For this review, take the finished solid that the model builds, in its own axes (mm). A direction names the side the tool comes from. Coordinates: 2 decimals unless noted, no trailing zeros. Order: outer loops, then holes, each group sorted by start corner. A loop starts at its lowest first (then second) coordinate and runs counter-clockwise, first axis right, second up. Notation, with made-up numbers: (81, -19) -> (138, -19) arc R33 cw to (138, 11) -> close; hole circle Ø2 at (65, 42.5). An arc over 180 degrees is marked (long way). Write item = value, one per line. Start each with the question number.
1) Insertion check: pin 1 Ø5 at (x, y) = (-81, 1) entering from -Z; pin 2 Ø3 at (y, z) = (27, 20) entering from +X; pin 3 Ø12.5 at (x, z) = (-18, 10) entering from +Y. Each pin has a flat end and moves straight along its axis. Give the tip position at first contact, or say it passes through.
2) Draft analysis for pull direction Z (two halves, no side actions). For faces 1 (the face through (-153.774, 16.355, 5.948)), 2 (the face through (-106.21, 14.37, 14.76)), 3 (the face through (12.697, -1.252, 12.979)), 4 (the face through (-49, -2.54, 13)), state which applies: +Z half, -Z half, draft (parallel to the pull), parting line (faces both ways), or undercut.
3) Machinability: for faces 5 (the face through (-153.61, 16.35, 21.36)), 6 (the face through (-103.632, 16, 17)), 7 (the face through (-71, -1, 0)), 8 (the face through (-108.712, 15, 10)), 9 (the face through (-156.11, 15.9, 22.45)), which of the approach directions +Z, -Z, +X, -X, +Y, -Y give a long, thin tool a straight path to every point of the face, cutting with its end or side? Answer none if there is none.
4) Consider section A-A on z = 3. Give the boundary of the cut face in (x, y), and give its area (3 significant figures).
5) Consider section C-C on x = -94. Give the boundary of the cut face in (y, z), and give its area (3 significant figures).
6) Wall thickness on probe 1 along Y at (x, z) = (-106.7, 12.7); probe 2 along X at (y, z) = (-1.15, 12.7); probe 3 along Y at (x, z) = (-83, 4.5): over which ranges is each line inside the solid? List them lowest first. Write a range as [from, to].
7) Consider section B-B on x = -131. Give the boundary of the cut face in (y, z), and give its area (3 significant figures).
from build123d import *

# Parameters (mm, degrees)
SKETCH1_R                   = 4.064
BOSS_EXTRUDE1_DEPTH         = 2.54
SKETCH2_W                   = 30.48
SKETCH2_H                   = 32.258
BOSS_EXTRUDE2_DEPTH         = 5.08
SKETCH3_W                   = 41.91
SKETCH3_H                   = 32.258
BOSS_EXTRUDE3_DEPTH         = 2.54
FILLET1_SIZE                = 2.54
CUT_EXTRUDE1_DEPTH          = 158.565599432
SKETCH5_W                   = 17.78
SKETCH5_H                   = 32.258
BOSS_EXTRUDE4_DEPTH         = 2.54
BOSS_EXTRUDE5_DEPTH         = 32.258
SKETCH9_W                   = 18.796
SKETCH9_H                   = 32.258
BOSS_EXTRUDE6_DEPTH         = 2.54
BOSS_EXTRUDE7_DEPTH         = 32.258
FILLET3_SIZE                = 2.54
W_0_22_DIAMETER_HOLE1_D     = 5.588
W_0_22_DIAMETER_HOLE1_DEPTH = 5.08
W_0_22_DIAMETER_HOLE1_TIP   = 1.67880457


with BuildPart() as part:
    # Sketch1 → Boss-Extrude1 (new body)
    with BuildSketch(Plane(origin=(0, 0, 0), x_dir=(1, 0, 0), z_dir=(0, 1, 0))):
        with BuildLine():
            Line((0, 0), (-108.712, 0))
            Line((-108.712, 0), (-108.712, -25.4))
            Line((-108.712, -25.4), (0, -25.4))
            ThreePointArc((0, -25.4), (12.7, -12.7), (0, 0))
        make_face()
        with Locations(Location((0, -12.7, 0), (0, 0, 270))):
            Circle(SKETCH1_R, mode=Mode.SUBTRACT)
    extrude(amount=-BOSS_EXTRUDE1_DEPTH)

    # Sketch2 → Boss-Extrude2 (add)
    with BuildSketch(Plane(origin=(-108.712, 0, 0), x_dir=(0, 0, -1), z_dir=(1, 0, 0))):
        with Locations((-15.24, 16.129)):
            Rectangle(SKETCH2_W, SKETCH2_H)
    extrude(amount=BOSS_EXTRUDE2_DEPTH)

    # Sketch3 → Boss-Extrude3 (add)
    with BuildSketch(Plane.XY.offset(30.48)):
        with Locations((-129.667, 16.129)):
            Rectangle(SKETCH3_W, SKETCH3_H)
    extrude(amount=-BOSS_EXTRUDE3_DEPTH)

    # Fillet1
    # a fillet whose section is not a circle: 2.54 mm, written as the material it adds along each edge
    with BuildSketch(Plane(origin=(-108.712, 0, 27.94), x_dir=(0, 0, -1), z_dir=(0, 1, 0))) as fillet1_piece_1:
        with BuildLine():
            Bezier((FILLET1_SIZE, 0), (0, 0), (0, FILLET1_SIZE), weights=[1, 1, 1])
            Line((0, FILLET1_SIZE), (0, 0))
            Line((0, 0), (FILLET1_SIZE, 0))
        make_face()
    extrude(amount=32.258)
    # a fillet whose section is not a circle: 2.54 mm, written as the material it takes off along each edge
    with BuildSketch(Plane(origin=(-103.632, -6.35, 30.48), x_dir=(0, 0, -1), z_dir=(0, 1, 0))) as fillet1_2_piece_1:
        with BuildLine():
            Bezier((FILLET1_SIZE, 0), (0, 0), (0, FILLET1_SIZE), weights=[1, 1, 1])
            Line((0, FILLET1_SIZE), (0, 0))
            Line((0, 0), (FILLET1_SIZE, 0))
        make_face()
    extrude(amount=44.958, mode=Mode.SUBTRACT)

    # Sketch4 → Cut-Extrude1 (cut, through all)
    with BuildSketch(Plane(origin=(0, 32.258, 0), x_dir=(1, 0, 0), z_dir=(0, 1, 0))):
        Polygon((-150.622, -27.94), (-148.082, -30.48), (-150.622, -30.48), align=None)
    extrude(amount=-CUT_EXTRUDE1_DEPTH, mode=Mode.SUBTRACT)



with BuildPart() as body_2:
    # Sketch5 → Boss-Extrude4 (new body)
    with BuildSketch(Plane(origin=(-89.281, 0, 89.281), x_dir=(0.7071067811865327, 0, 0.7071067811865624), z_dir=(-0.7071067811865624, 0, 0.7071067811865327))):
        with Locations((-95.63927413, 16.129)):
            Rectangle(SKETCH5_W, SKETCH5_H)
    extrude(amount=-BOSS_EXTRUDE4_DEPTH)


with BuildPart() as part_1:
    add(part.part)

    add(body_2.part)  # Boss-Extrude5 merges body 2
    # Sketch6 → Boss-Extrude5 (add)
    with BuildSketch(Plane(origin=(0, 32.258, 0), x_dir=(1, 0, 0), z_dir=(0, 1, 0))):
        Polygon((-150.622, -27.94), (-147.029897552, -27.94), (-148.825948776, -26.143948776), align=None)
    extrude(amount=-BOSS_EXTRUDE5_DEPTH)

    # Fillet2
    # a fillet whose section is not a circle: 2.54 mm, written as the material it adds along each edge
    with BuildSketch(Plane(origin=(-147.029897552, 32.258, 27.94), x_dir=(-0.7071067811865357, 0, -0.7071067811865592), z_dir=(0, -1, 0))) as fillet2_piece_1:
        with BuildLine():
            Bezier((1.052102448, 0), (0, 0), (-0.743948776, 0.743948776), weights=[1, 1, 1])
            Line((-0.743948776, 0.743948776), (0, 0))
            Line((0, 0), (1.052102448, 0))
        make_face()
    extrude(amount=32.258)
    # a fillet whose section is not a circle: 2.54 mm, written as the material it takes off along each edge
    with BuildSketch(Plane(origin=(-148.082, 34.888256121, 30.48), x_dir=(-0.707106781186539, 0, -0.707106781186556), z_dir=(0, -1, 0))) as fillet2_2_piece_1:
        with BuildLine():
            Bezier((1.052102448, 0), (0, 0), (-0.743948776, 0.743948776), weights=[1, 1, 1])
            Line((-0.743948776, 0.743948776), (0, 0))
            Line((0, 0), (1.052102448, 0))
        make_face()
    extrude(amount=37.518512242, mode=Mode.SUBTRACT)



with BuildPart() as body_2_2:
    # Sketch9 → Boss-Extrude6 (new body)
    with BuildSketch(Plane(origin=(-73.913358569, 0, -73.913358569), x_dir=(-0.7071067811865623, 0, 0.7071067811865328), z_dir=(-0.7071067811865328, 0, -0.7071067811865623))):
        with Locations((114.324401062, 16.129)):
            Rectangle(SKETCH9_W, SKETCH9_H)
    extrude(amount=BOSS_EXTRUDE6_DEPTH)


with BuildPart() as part_2:
    add(part_1.part)

    add(body_2_2.part)  # Boss-Extrude7 merges body 2 2
    # Sketch10 → Boss-Extrude7 (add)
    with BuildSketch(Plane(origin=(0, 0, 0), x_dir=(1, 0, 0), z_dir=(0, 1, 0))):
        Polygon((-161.398307345, -13.571590206), (-163.194358569, -11.775538982), (-164.990409794, -13.571590206), (-163.194358569, -15.367641431), align=None)
    extrude(amount=BOSS_EXTRUDE7_DEPTH)

    # Fillet3
    # a fillet whose section is not a circle: 2.54 mm, written as the material it adds along each edge
    with BuildSketch(Plane(origin=(-161.398307345, 32.258, 13.571590206), x_dir=(0.7071067811865611, 0, -0.7071067811865339), z_dir=(0, -1, 0))) as fillet3_piece_1:
        with BuildLine():
            Bezier((FILLET3_SIZE, 0), (0, 0), (0, FILLET3_SIZE), weights=[1, 1, 1])
            Line((0, FILLET3_SIZE), (0, 0))
            Line((0, 0), (FILLET3_SIZE, 0))
        make_face()
    extrude(amount=32.258)
    # a fillet whose section is not a circle: 2.54 mm, written as the material it takes off along each edge
    with BuildSketch(Plane(origin=(-164.990409794, -6.35, 13.571590206), x_dir=(0.7071067811865199, 0, 0.7071067811865752), z_dir=(0, 1, 0))) as fillet3_2_piece_1:
        with BuildLine():
            Bezier((FILLET3_SIZE, 0), (0, 0), (0, FILLET3_SIZE), weights=[1, 1, 1])
            Line((0, FILLET3_SIZE), (0, 0))
            Line((0, 0), (FILLET3_SIZE, 0))
        make_face()
    extrude(amount=44.958, mode=Mode.SUBTRACT)

    # W (0.22) Diameter Hole1
    with Locations(Plane(origin=(-103.632, 16.256, 12.7), x_dir=(0, 0, 1), z_dir=(1, 0, 0))):
        with Locations((0, 0)):
            Hole(W_0_22_DIAMETER_HOLE1_D / 2, depth=W_0_22_DIAMETER_HOLE1_DEPTH)
            with Locations((0, 0, -(W_0_22_DIAMETER_HOLE1_DEPTH + W_0_22_DIAMETER_HOLE1_TIP / 2))):  # 118° drill point
                Cone(0, W_0_22_DIAMETER_HOLE1_D / 2, W_0_22_DIAMETER_HOLE1_TIP, mode=Mode.SUBTRACT)


solid = part_2.part
Answer sheet:
q1.pin_1 = 0
q1.pin_2 = -103.63
q1.pin_3 = 0
q2.face_1 = undercut
q2.face_2 = undercut
q2.face_3 = parting line
q2.face_4 = draft
q3.face_5 = +Y, -Y
q3.face_6 = +Z, -Z, +X, +Y
q3.face_7 = -Z, +X, +Y, -Y
q3.face_8 = -Z, +Y, -Y
q3.face_9 = +Z, -X, +Y, -Y
q4.outline = (-154.42, 0) -> (-150.83, 0) -> (-150.83, 32.26) -> (-154.42, 32.26) -> close; (-108.71, -2.54) -> (8.2, -2.54) -> (8.2, 0) -> (-103.63, 0) -> (-103.63, 32.26) -> (-108.71, 32.26) -> close
q4.area = 577 mm2
q5.outline = (-2.54, 0) -> (0, 0) -> (0, 25.4) -> (-2.54, 25.4) -> close
q5.area = 64.5 mm2
q6.probe_1 = [-2.54, 13.46], [19.05, 32.26]
q6.probe_2 = [-108.71, -4.06], [4.06, 12.7]
q6.probe_3 = [-2.54, 0]
q7.outline = (0, 27.94) -> (32.26, 27.94) -> (32.26, 30.48) -> (0, 30.48) -> close
q7.area = 81.9 mm2
